Design review of the part built by this model. Coordinates are the model's own, in mm. A direction names the side the tool comes from. Give positions to 0.01 mm unless a question says otherwise; leave off trailing zeros. Write each loop counter-clockwise with the first axis right and the second up, starting at its lowest first coordinate (ties: lowest second). Pieces come first, ordered by that corner, then holes. Notation, with made-up numbers: (23.25, -32.75) -> (30.25, -32.75) arc R24 ccw to (30.25, 4.25) -> close; hole circle Ø5 at (-13, 63). An arc over 180 degrees is marked (long way). Answer as a JSON object with one key per item and string values.
```python
from build123d import *

# Parameters (mm, degrees)
BOSS_EXTRUDE1_DEPTH = 71.12
SKETCH4_W           = 9.4615
SKETCH4_H           = 3.175
CUT_EXTRUDE1_DEPTH  = 72.12
BOSS_EXTRUDE2_DEPTH = 71.12
FILLET2_R           = 6.35
FILLET4_R           = 1.27
SKETCH6_W           = 101.6
SKETCH6_H           = 71.12
BOSS_EXTRUDE3_DEPTH = 3.175
SKETCH7_R           = 2.0193
CUT_EXTRUDE2_DEPTH  = 80.4385
SKETCH8_R           = 2.0193
CUT_EXTRUDE3_DEPTH  = 42.275
SKETCH9_R           = 3.96875
CUT_EXTRUDE4_DEPTH  = 42.275
FILLET5_R           = 2.54
SKETCH10_R          = 5.08
CUT_EXTRUDE5_DEPTH  = 3.175


with BuildPart() as part:
    # Sketch3 → Boss-Extrude1 (new body)
    with BuildSketch(Plane.XY):
        with BuildLine():
            Line((0, 6.35), (0, 33.655))
            ThreePointArc((0, 33.655), (-0.371974388, 34.553025612), (-1.27, 34.925))
            Line((-1.27, 34.925), (-3.175, 34.925))
            Line((-3.175, 34.925), (-3.175, 0))
            Line((-3.175, 0), (-3.175, -3.175))
            Line((-3.175, -3.175), (34.925, -3.175))
            Line((34.925, -3.175), (34.925, -1.27))
            ThreePointArc((34.925, -1.27), (34.553025612, -0.371974388), (33.655, 0))
            Line((33.655, 0), (6.35, 0))
            ThreePointArc((6.35, 0), (1.859871939, 1.859871939), (0, 6.35))
        make_face()
    extrude(amount=BOSS_EXTRUDE1_DEPTH)

    # Sketch4 → Cut-Extrude1 (cut, through all)
    with BuildSketch(Plane(origin=(0, 0, 0), x_dir=(-1, 0, 0), z_dir=(0, 0, -1))):
        with Locations((-30.19425, -1.5875)):
            Rectangle(SKETCH4_W, SKETCH4_H)
    extrude(amount=-CUT_EXTRUDE1_DEPTH, mode=Mode.SUBTRACT)

    # Sketch5 → Boss-Extrude2 (add)
    with BuildSketch(Plane(origin=(0, 0, 0), x_dir=(-1, 0, 0), z_dir=(0, 0, -1))):
        Polygon((-25.4635, -3.175), (-54.102, -3.175), (-54.102, 34.925), (-50.927, 34.925), (-50.927, 0), (-25.4635, 0), align=None)
    extrude(amount=-BOSS_EXTRUDE2_DEPTH)

    # Fillet2
    fillet2_edges = [part.edges().sort_by_distance(p)[0] for p in [
        (50.927, 0, 35.56),
    ]]
    fillet(fillet2_edges, radius=FILLET2_R)

    # Fillet4
    fillet4_edges = [part.edges().sort_by_distance(p)[0] for p in [
        (50.927, 34.925, 35.56),
    ]]
    fillet(fillet4_edges, radius=FILLET4_R)

    # Sketch6 → Boss-Extrude3 (add)
    with BuildSketch(Plane.XZ.offset(3.175)):
        with Locations((25.4635, 35.56)):
            Rectangle(SKETCH6_W, SKETCH6_H)
    extrude(amount=BOSS_EXTRUDE3_DEPTH)

    # Sketch7 → Cut-Extrude2 (cut, through all)
    with BuildSketch(Plane.ZY.offset(3.175)):
        with Locations((16.51, 25.146)):
            Circle(SKETCH7_R)
        with Locations((54.61, 25.146)):
            Circle(SKETCH7_R)
    extrude(amount=-CUT_EXTRUDE2_DEPTH, mode=Mode.SUBTRACT)

    # Sketch8 → Cut-Extrude3 (cut, through all)
    with BuildSketch(Plane.XZ.offset(6.35)):
        with Locations((25.4635, 16.51)):
            Circle(SKETCH8_R)
        with Locations((25.4635, 54.61)):
            Circle(SKETCH8_R)
    extrude(amount=-CUT_EXTRUDE3_DEPTH, mode=Mode.SUBTRACT)

    # Sketch9 → Cut-Extrude4 (cut, through all)
    with BuildSketch(Plane.XZ.offset(6.35)):
        with Locations((-15.8115, 16.51)):
            Circle(SKETCH9_R)
        with Locations((-15.8115, 54.61)):
            Circle(SKETCH9_R)
        with Locations((66.7385, 54.61)):
            Circle(SKETCH9_R)
        with Locations((66.7385, 16.51)):
            Circle(SKETCH9_R)
    extrude(amount=-CUT_EXTRUDE4_DEPTH, mode=Mode.SUBTRACT)

    # Fillet5
    fillet5_edges = [part.edges().sort_by_distance(p)[0] for p in [
        (-3.175, -3.175, 35.56),
        (54.102, -3.175, 35.56),
    ]]
    fillet(fillet5_edges, radius=FILLET5_R)

    # Sketch10 → Cut-Extrude5 (cut)
    with BuildSketch(Plane.XZ.offset(6.35)):
        with Locations((25.4635, 54.61)):
            Circle(SKETCH10_R)
        with Locations((25.4635, 16.51)):
            Circle(SKETCH10_R)
    extrude(amount=-CUT_EXTRUDE5_DEPTH, mode=Mode.SUBTRACT)


solid = part.part
```
(1) We need section C-C, the plane x = 33. State the section outline as (y, z) points, then the cut area to 3 significant figures.
Here are the results:
{"outline": "(-6.35, 0) -> (0, 0) -> (0, 71.12) -> (-6.35, 71.12) -> close", "area": "452 mm²"}
(2) We need section B-B, the plane z = 16.51. Give the number of separate pieces and of enclosed holes in the cut face, then the cut area to 3 significant figures.
Here are the results:
{"separate pieces": "6", "enclosed holes": "0", "area": "624 mm²"}
(3) We need section D-D, the plane x = -9. State the section outline as (y, z) points (3 decimals).
Here are the results:
{"outline": "(-6.35, 0) -> (-3.175, 0) -> (-3.175, 71.12) -> (-6.35, 71.12) -> close"}
(4) For faces 1 (the cylindrical face through (49.017, 1.811, 36.058)), 2 (the flat face through (-16, -3.175, 36)), 3 (the flat face through (66, -3.175, 36)), 4 (the flat face through (25, -1, 71.12)), 5 (the cylindrical face through (30.309, -4.785, 18.036)), list the 3-axis set-ups (+Z, -Z, +X, -X, +Y, -Y) from which the entire face can be reached by the end or side of a thin tool; tool diameter is ignored.
Here are the results:
{"face 1": "+Z, -Z, +Y", "face 2": "+Z, -Z, -X, +Y", "face 3": "+Z, -Z, +X, +Y", "face 4": "+Z, +X, -X, +Y, -Y", "face 5": "-Y"}
(5) For line 1 along X through (y, z) = (22.5, 8.5) (3 decimals); line 2 along Z through (x, y) = (-2.5, 24); line 3 along Y through (x, z) = (42, 56), list the stretches that pass through material, from the lowest coordinate up.
Here are the results:
{"line 1": "x = -3.175 to 0, 50.927 to 54.102", "line 2": "z = 0 to 14.85, 18.17 to 52.95, 56.27 to 71.12", "line 3": "y = -6.35 to 0"}
(6) Clearance check with flat-ended pins moving along their axes: pin 1 (3.5 mm diameter, centred on x = 25.46, z = 54.61, fed in from +Y); pin 2 (10 mm diameter, centred on x = 66, z = 19, fed in from +Y) (3 decimals); pin 3 (5.5 mm diameter, centred on y = 25.146, z = 54.61, fed in from -X) (3 decimals); pin 4 (3 mm diameter, centred on x = 24, z = 16.5, fed in from -Y) (3 decimals). State where each tip first meets the part, or that it passes through.
Here are the results:
{"pin 1": "passes through", "pin 2": "stops at y = -3.175", "pin 3": "stops at x = -3.175", "pin 4": "stops at y = -3.175"}
(7) The part is to be moulded in two halves that separate along Z. For faces 6 (the cylindrical face through (63.81, -4.78, 19.19)), 7 (the flat face through (-25.336, -5, 35)), 8 (the flat face through (25, -1, 0)), say which applies: +Z half, -Z half, draft (parallel to the pull), parting line (faces both ways), or undercut.
Here are the results:
{"face 6": "undercut", "face 7": "draft", "face 8": "-Z half"}
